Read the model definition and answer for the solid it produces. Units are mm, in the model's axes. A direction names the side the tool comes from. Round coordinates to 2 decimals unless told otherwise and drop trailing zeros. Loops run counter-clockwise (first coordinate to the right, second up) from the corner with the lowest first, then second, coordinate; pieces in that order, holes last. Notation, with made-up numbers: (83.5, -36.75) -> (127.5, -36.75) arc R28 ccw to (127.5, -15.75) -> close; hole circle Ø9 at (4.5, 84). An arc over 180 degrees is marked (long way). Put each result on its own line as item: value.
from build123d import *

# Parameters (mm, degrees)
SKETCH_2_R          = 21.1
SKETCH_2_R_2        = 15.1
SKETCH_2_R_3        = 1.6
EXTRUDE_1_DEPTH     = 3
SKETCH_4_R          = 3
CUT_EXTRUDE_1_DEPTH = 3
SKETCH_5_R          = 4
CUT_EXTRUDE_2_DEPTH = 42
EXTRUDE_4_DEPTH     = 2.5


with BuildPart() as part:
    # 草图1 → 旋转1 (revolve)
    with BuildSketch(Plane.XY, mode=Mode.PRIVATE) as revolve_1_sk:
        Polygon((12.1, -0.34341598), (12.1, 4.65658402), (10.1, 4.65658402), (10.1, 34.65658402), (12.1, 34.65658402), (12.1, 39.65658402), (15.1, 39.65658402), (15.1, -0.34341598), align=None)
    revolve(revolve_1_sk.sketch.rotate(Axis((0, 0, 0), (0, 1, 0)), 90), axis=Axis((0, 0, 0), (0, 1, 0)))

    # 草图2 → 凸台-拉伸1 (add)
    with BuildSketch(Plane.XZ.offset(0.34341598)):
        with Locations(Location((0, 0, 0), (0, 0, 270))):
            Circle(SKETCH_2_R)
        with Locations(Location((0, 0, 0), (0, 0, 270))):
            Circle(SKETCH_2_R_2, mode=Mode.SUBTRACT)
        with Locations(Location((-12.798632739, 12.798632739, 0), (0, 0, 270))):
            Circle(SKETCH_2_R_3, mode=Mode.SUBTRACT)
        with Locations(Location((12.798632739, 12.798632739, 0), (0, 0, 270))):
            Circle(SKETCH_2_R_3, mode=Mode.SUBTRACT)
        with Locations(Location((12.798632739, -12.798632739, 0), (0, 0, 270))):
            Circle(SKETCH_2_R_3, mode=Mode.SUBTRACT)
        with Locations(Location((-12.798632739, -12.798632739, 0), (0, 0, 270))):
            Circle(SKETCH_2_R_3, mode=Mode.SUBTRACT)
    extrude(amount=-EXTRUDE_1_DEPTH)

    # 草图4 → 切除-拉伸1 (cut)
    with BuildSketch(Plane.XZ.offset(0.34341598)):
        with Locations((0, 20)):
            Circle(SKETCH_4_R)
        with Locations((17.320508076, -10)):
            Circle(SKETCH_4_R)
        with Locations((-17.320508076, -10)):
            Circle(SKETCH_4_R)
    extrude(amount=-CUT_EXTRUDE_1_DEPTH, mode=Mode.SUBTRACT)

    # 草图5 → 切除-拉伸2 (cut)
    with BuildSketch(Plane.XY):
        with Locations(Location((0, 13.65658402, 0), (0, 0, 270))):
            Circle(SKETCH_5_R)
    extrude(amount=-CUT_EXTRUDE_2_DEPTH, mode=Mode.SUBTRACT)

    # 草图6 → 凸台-拉伸4 (add)
    with BuildSketch(Plane(origin=(0, 39.65658402, 0), x_dir=(1, 0, 0), z_dir=(0, 1, 0))):
        with BuildLine():
            Line((12.458840363, 4.048122626), (14.360953396, 4.666156615))
            ThreePointArc((14.360953396, 4.666156615), (0, 15.1), (-14.360953396, 4.666156615))
            Line((-14.360953396, 4.666156615), (-12.458840363, 4.048122626))
            ThreePointArc((-12.458840363, 4.048122626), (0, 13.1), (12.458840363, 4.048122626))
        make_face()
    extrude(amount=EXTRUDE_4_DEPTH)


solid = part.part
Item 1: For a pull along X with two mould halves and no side action, classify faces 1 (the cylindrical face through (-18.14, 1.14, 10.78)), 2 (the cylindrical face through (-0.27, 1.14, -21.1)), 3 (the cylindrical face through (0, 1, 17)), 4 (the flat face through (13.397, 40.889, -4.353)) as pulls with the +X half, pulls with the -X half, needs draft (parallel to the pull), parting line crosses it, or undercut.
Derived:
face 1: pulls with the -X half
face 2: parting line crosses it
face 3: undercut
face 4: pulls with the +X half
Item 2: The part is cut by section A-A (z = 0). Determine the outline of the cut face in (x, y), then the cut area to 3 significant figures.
Derived:
outline: (-21.1, -0.34) -> (-12.1, -0.34) -> (-12.1, 4.66) -> (-10.1, 4.66) -> (-10.1, 34.66) -> (-12.1, 34.66) -> (-12.1, 39.66) -> (-15.1, 39.66) -> (-15.1, 2.66) -> (-21.1, 2.66) -> close; (10.1, 4.66) -> (12.1, 4.66) -> (12.1, -0.34) -> (21.1, -0.34) -> (21.1, 2.66) -> (15.1, 2.66) -> (15.1, 39.66) -> (12.1, 39.66) -> (12.1, 34.66) -> (10.1, 34.66) -> close
area: 396 mm^2
Item 3: Flat-ended cylindrical pins translate along their axes: pin 1 Ø12 at (y, z) = (31, 1) entering from +X; pin 2 Ø8 at (x, y) = (-2, 16) entering from -Z; pin 3 Ø10 at (x, z) = (4.5, 5) entering from -Y. Find the tip coordinate at first contact, or state that the pin passes through.
Derived:
pin 1: stops at x = 15.1
pin 2: stops at z = -15.1
pin 3: stops at y = 4.66
Item 4: Find the intervals of material crossed by line 1 along X through (y, z) = (14, 0); line 2 along Z through (x, y) = (0.5, 32); line 3 along X through (y, z) = (0.95, 0), in increasing order.
Derived:
line 1: x = -15.1 to -10.1, 10.1 to 15.1
line 2: z = -15.09 to -10.09, 10.09 to 15.09
line 3: x = -21.1 to -12.1, 12.1 to 21.1
Item 5: The part is cut by section D-D (z = 18). Determine the outline of the cut face in (x, y).
Derived:
outline: (-11.01, -0.34) -> (-2.24, -0.34) -> (-2.24, 2.66) -> (-11.01, 2.66) -> close; (2.24, -0.34) -> (11.01, -0.34) -> (11.01, 2.66) -> (2.24, 2.66) -> close
Item 6: Which of the six approach directions +Z, -Z, +X, -X, +Y, -Y give full straight-line access (tool end or side, diameter ignored) to faces 5 (the cylindrical face through (-3.635, 2.192, -11.541)), 6 (the flat face through (14.2, 2.657, 6.2)), 7 (the flat face through (-13.42, 40.89, -4.36)), 8 (the cylindrical face through (-1.53, 9.96, -12.15))?
Derived:
face 5: -Y
face 6: +Y
face 7: +Z, -X, +Y
face 8: -Z
Item 7: The part is cut by section B-B (x = 0). Determine the outline of the cut face in (y, z).
Derived:
outline: (-0.34, -21.1) -> (2.66, -21.1) -> (2.66, -15.1) -> (9.66, -15.1) -> (9.66, -10.1) -> (4.66, -10.1) -> (4.66, -12.1) -> (-0.34, -12.1) -> close; (-0.34, 12.1) -> (4.66, 12.1) -> (4.66, 10.1) -> (34.66, 10.1) -> (34.66, 12.1) -> (39.66, 12.1) -> (39.66, 15.1) -> (2.66, 15.1) -> (2.66, 17) -> (-0.34, 17) -> close; (17.66, -15.1) -> (42.16, -15.1) -> (42.16, -13.1) -> (39.66, -13.1) -> (39.66, -12.1) -> (34.66, -12.1) -> (34.66, -10.1) -> (17.66, -10.1) -> close
Item 8: The part is cut by section C-C (y = 24). Determine the outline of the cut face in (x, z), then the cut area to 3 significant figures.
Derived:
outline: circle Ø30.2 at (0, 0); hole circle Ø20.2 at (0, 0)
area: 396 mm^2
